The listing builds one solid part. Answer for the finished solid, in the listing's coordinates (mm). Coordinates: 2 decimals unless noted, no trailing zeros. Write each loop counter-clockwise with the first axis right and the second up, starting at its lowest first coordinate (ties: lowest second). Pieces come first, ordered by that corner, then holes.
from build123d import *

# Parameters (mm, degrees)
F1_DEPTH = 1060
F2_R     = 2
F4_DEPTH = 40.001


with BuildPart() as f1:
    # F0 (on Front) → F1 (new body)
    with BuildSketch(Plane.XZ):
        Polygon((0, 40), (0, 0), (32.190853, 0), (50, 40), align=None)
    extrude(amount=F1_DEPTH)

    # F2
    f2_edges = [f1.edges().sort_by_distance(p)[0] for p in [
        (50, -530, 40),
    ]]
    fillet(f2_edges, radius=F2_R)

    # F3 (on face) → F4 (cut, through all)
    with BuildSketch(Plane.XY.offset(40)):
        Polygon((49.361777, 0), (0, 0), (49.361777, -49.361777), align=None)
        Polygon((60.1357, -999.8643), (0, -1060), (60.1357, -1060), align=None)
    extrude(amount=-F4_DEPTH, mode=Mode.SUBTRACT)


solid = f1.part
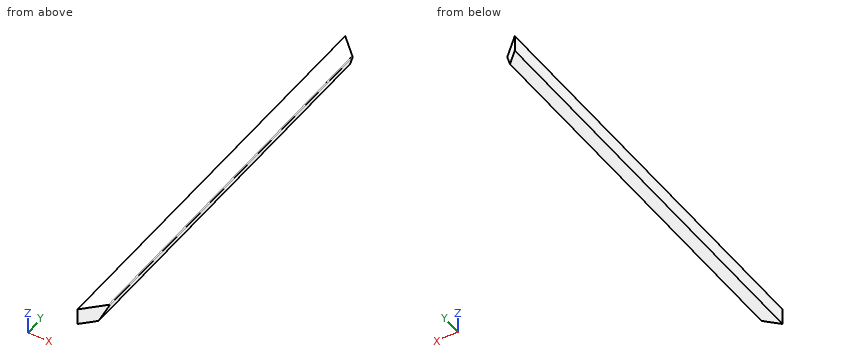
1. Section A-A on y = -302.5 is taken. Give the vertices of the cut face in (x, z).
Results found:
outline: (0, 0) - (32.19, 0) - (48.75, 37.19) arc R2 ccw to (46.92, 40) - (0, 40) - close
2. Section B-B on x = 22 is taken. Give the vertices of the cut face in (y, z), then the cut area to 3 significant figures.
Results found:
outline: (-1038, 0) - (-22, 0) - (-22, 40) - (-1038, 40) - close
area: 40,600 mm2
3. Flat-ended cylindrical pins translate along their axes: P1, Ø3, axis at x = 26.5, z = 27.5, coming from the +Y side; P2, Ø1.5, axis at y = -854, z = 17, coming from the +X side; P3, Ø1.5, axis at x = 5.5, z = 19.5, coming from the -Y side. Find the tip coordinate at first contact, or state that the pin passes through.
Results found:
P1: stops at y = -25
P2: stops at x = 40.09
P3: stops at y = -1055.25
4. Section C-C on z = 18.5 is taken. Give the vertices of the cut face in (x, y), then the cut area to 3 significant figures.
Results found:
outline: (0, -1060) - (40.43, -1019.57) - (40.43, -40.43) - (0, 0) - close
area: 41,200 mm2
5. Find the intervals of material crossed by L1, parallel to X at y = -196.5, z = 37.5; L2, parallel to X at y = -945.5, z = 11; L3, parallel to Z at x = 46.5, y = -461, in increasing order.
Results found:
L1: x = 0 to 48.86
L2: x = 0 to 37.09
L3: z = 32.14 to 40
